Check sheet for the modelled part. Datum: model origin and axes. Units: mm. A direction names the side the tool comes from. Round coordinates to 2 decimals unless told otherwise and drop trailing zeros. Loops run counter-clockwise (first coordinate to the right, second up) from the corner with the lowest first, then second, coordinate; pieces in that order, holes last. Notation, with made-up numbers: (53, -17) - (68, -17) arc R9 ccw to (68, -7) - close; hole circle Ø3 at (44.25, 87.5). An arc over 180 degrees is marked (long way). Answer in a Markdown table with one row per item. Add a question column.
(1) Cross-section at C-C on y = 24.89. Enter the section's corners in (x, z), then the cut area to 3 significant figures.
(2) Thickness scan on line 1 along Y through (x, z) = (5, 6.5); line 2 along X through (y, z) = (13, 8.25); line 3 along X through (y, z) = (-54.5, 8.75). Record the ranges inside material, lowest first.
(3) Cross-section at B-B on x = 2.5. Enter the section's corners in (y, z), then the cut area to 3 significant figures.
(4) Access from +Z, -Z, +X, -X, +Y, -Y to the whole of each face (thin tool, end or side, straight path). Record for faces 1 (the flat face through (-3, -27.3, 5)), 2 (the flat face through (19, -15, 7.34)), 3 (the flat face through (23.813, -15, 5)), 4 (the flat face through (0, -20.3, 5)), 5 (the flat face through (18, -59.002, 4)).
(5) Mould release check, pull along Y, two halves, no side actions. Record for faces 6 (the flat face through (11, -6, 10.46)), 7 (the flat face through (4, 27.3, 5)), 8 (the cylindrical face through (4.87, 25.88, 5.3)): +Y half, -Y half, draft (parallel to the pull), parting line (faces both ways), or undercut.
(6) Gauge pin test, flat ends, axial feed: pin 1 (1.5 mm diameter, centred on y = -32.5, z = 7.5, fed in from -X); pin 2 (2.5 mm diameter, centred on x = 5, y = -24.9, fed in from -Z); pin 3 (4 mm diameter, centred on x = -10, z = 3.5, fed in from -Y); pin 4 (1.6 mm diameter, centred on x = 5, y = 24.89, fed in from -Z). Record the tip position at first contact, or that the pin passes through.
(7) Cross-section at A-A on z = 9.5. Enter the section's corners in (x, y).
(8) Cross-section at D-D on y = -6. Enter the section's corners in (x, z), then the cut area to 3 significant figures.
from build123d import *

# Parameters (mm, degrees)
BOSS_EXTRUDE2_DEPTH = 10.46
CUT_EXTRUDE1_DEPTH  = 3.12
SKETCH5_R           = 1
CUT_EXTRUDE2_DEPTH  = 20


with BuildPart() as part:
    # Sketch2 → Boss-Extrude2 (new body)
    with BuildSketch(Plane.XY):
        Polygon((-7.9, 27.3), (23.813102619, 27.3), (23.813102619, -59.002149985), (11.813102619, -59.002149985), (11.813102619, -27.3), (-2.175, -27.3), (-16.9, -27.3), (-16.9, 27.3), align=None)
        Polygon((-9.9, -20.3), (9.9, -20.3), (9.9, -19.3), (9.9, 20.3), (-9.9, 20.3), align=None, mode=Mode.SUBTRACT)
    extrude(amount=BOSS_EXTRUDE2_DEPTH)

    # Sketch4 → Cut-Extrude1 (cut)
    with BuildSketch(Plane.XY.offset(10.46)):
        Polygon((17.813102619, -59.002149985), (17.2, -59.002149985), (16.150910181, -59.002149985), (16.150910181, 27.3), (17.2, 27.3), (22.113102619, 27.3), (22.113102619, -59.002149985), align=None)
    extrude(amount=-CUT_EXTRUDE1_DEPTH, mode=Mode.SUBTRACT)

    # Sketch5 → Cut-Extrude2 (cut)
    with BuildSketch(Plane.XY.offset(10.46)):
        with Locations((-5, -24.9)):
            Circle(SKETCH5_R)
        with Locations((5, -24.9)):
            Circle(SKETCH5_R)
        with Locations((-5, 24.89)):
            Circle(SKETCH5_R)
        with Locations((5, 24.89)):
            Circle(SKETCH5_R)
    extrude(amount=-CUT_EXTRUDE2_DEPTH, mode=Mode.SUBTRACT)


solid = part.part
Answers:
| question | item | result |
|---|---|---|
| 1 | outline | (-16.9, 0) - (-6, 0) - (-6, 10.46) - (-16.9, 10.46) - close; (-4, 0) - (4, 0) - (4, 10.46) - (-4, 10.46) - close; (6, 0) - (23.81, 0) - (23.81, 10.46) - (22.11, 10.46) - (22.11, 7.34) - (16.15, 7.34) - (16.15, 10.46) - (6, 10.46) - close |
| 1 | area | 365 mm^2 |
| 2 | line 1 | y = -27.3 to -25.9, -23.9 to -20.3, 20.3 to 23.89, 25.89 to 27.3 |
| 2 | line 2 | x = -16.9 to -9.9, 9.9 to 16.15, 22.11 to 23.81 |
| 2 | line 3 | x = 11.81 to 16.15, 22.11 to 23.81 |
| 3 | outline | (-27.3, 0) - (-20.3, 0) - (-20.3, 10.46) - (-27.3, 10.46) - close; (20.3, 0) - (27.3, 0) - (27.3, 10.46) - (20.3, 10.46) - close |
| 3 | area | 146 mm^2 |
| 4 | face 1 | +Z, -Z, -X, -Y |
| 4 | face 2 | +Z, +Y, -Y |
| 4 | face 3 | +Z, -Z, +X, +Y, -Y |
| 4 | face 4 | +Z, -Z |
| 4 | face 5 | +Z, -Z, +X, -X, -Y |
| 5 | face 6 | draft |
| 5 | face 7 | +Y half |
| 5 | face 8 | undercut |
| 6 | pin 1 | stops at x = 11.81 |
| 6 | pin 2 | stops at z = 0 |
| 6 | pin 3 | stops at y = -27.3 |
| 6 | pin 4 | passes through |
| 7 | outline | (-16.9, -27.3) - (11.81, -27.3) - (11.81, -59) - (16.15, -59) - (16.15, 27.3) - (-16.9, 27.3) - close; (22.11, -59) - (23.81, -59) - (23.81, 27.3) - (22.11, 27.3) - close; hole (-9.9, -20.3) - (9.9, -20.3) - (9.9, 20.3) - (-9.9, 20.3) - close; hole circle Ø2 at (-5, -24.9); hole circle Ø2 at (-5, 24.89); hole circle Ø2 at (5, -24.9); hole circle Ø2 at (5, 24.89) |
| 8 | outline | (-16.9, 0) - (-9.9, 0) - (-9.9, 10.46) - (-16.9, 10.46) - close; (9.9, 0) - (23.81, 0) - (23.81, 10.46) - (22.11, 10.46) - (22.11, 7.34) - (16.15, 7.34) - (16.15, 10.46) - (9.9, 10.46) - close |
| 8 | area | 200 mm^2 |
